from build123d import *

# Parameters (mm, degrees)
F0_R      = 9.1
F1_DEPTH  = 20
F2_W      = 10
F2_H      = 17
F3_DEPTH  = 30
F4_W      = 10
F4_H      = 28
F5_DEPTH  = 25.4
F6_R      = 3
F7_R      = 1.99999
F8_R      = 2.5527
F9_DEPTH  = 7.001
F10_R     = 1.35255
F11_DEPTH = 3.6831519111


# Not quite as in the source:
# - a fillet or chamfer is up to 0.001 mm smaller than in the source, because OpenCascade refuses the exact size


with BuildPart() as f1:
    # F0 (on Top) → F1 (new body)
    with BuildSketch(Plane.XY):
        with BuildLine():
            ThreePointArc((2.8507034294, -10.1056167529), (8.3720483159, -6.3370976792), (10.5, 0))
            ThreePointArc((10.5, 0), (9.0208092763, 5.3735463151), (5, 9.2330926563))
            Line((5, 9.2330926563), (-5, 9.2330926563))
            ThreePointArc((-5, 9.2330926563), (-10.4357465707, -1.1598247764), (-2.8507034294, -10.1056167529))
            Line((-2.8507034294, -10.1056167529), (2.8507034294, -10.1056167529))
        make_face()
        Circle(F0_R, mode=Mode.SUBTRACT)
        with BuildLine():
            Line((-5, 9.2330926563), (5, 9.2330926563))
            ThreePointArc((5, 9.2330926563), (0, 10.5), (-5, 9.2330926563))
        make_face()
        with BuildLine():
            ThreePointArc((-5, 9.2330926563), (0, 10.5), (5, 9.2330926563))
            Line((5, 9.2330926563), (5, 26.2330926563))
            Line((5, 26.2330926563), (-5, 26.2330926563))
            Line((-5, 26.2330926563), (-5, 9.2330926563))
        make_face()
        with BuildLine():
            Line((2.8507034294, -12.6810744405), (2.8507034294, -10.1056167529))
            ThreePointArc((2.8507034294, -10.1056167529), (0, -10.5), (-2.8507034294, -10.1056167529))
            Line((-2.8507034294, -10.1056167529), (-2.8507034294, -12.6810744405))
            Line((-2.8507034294, -12.6810744405), (2.8507034294, -12.6810744405))
        make_face()
        with BuildLine():
            ThreePointArc((-2.8507034294, -10.1056167529), (0, -10.5), (2.8507034294, -10.1056167529))
            Line((2.8507034294, -10.1056167529), (-2.8507034294, -10.1056167529))
        make_face()
    extrude(amount=F1_DEPTH)

    # F2 (on face) → F3 (join)
    with BuildSketch(Plane.XY.offset(20)):
        with Locations((0, 17.7330926563)):
            Rectangle(F2_W, F2_H)
    extrude(amount=F3_DEPTH)

    # F4 (on face) → F5 (cut)
    with BuildSketch(Plane.YZ.offset(5)):
        with Locations((14.2330926563, 36)):
            Rectangle(F4_W, F4_H)
    extrude(amount=-F5_DEPTH, mode=Mode.SUBTRACT)

    # F6
    f6_edges = [f1.edges().sort_by_distance(p)[0] for p in [
        (5, 9.233093, 10),
        (-5, 9.233093, 10),
        (-5, 22.733093, 50),
        (5, 22.733093, 50),
        (2.850703, -10.105617, 10),
        (-2.850703, -10.105617, 10),
    ]]
    fillet(f6_edges, radius=F6_R)

    # F7 (radius 2 in the source; OpenCascade refuses exactly that, so slightly less here)
    f7_edges = [f1.edges().sort_by_distance(p)[0] for p in [
        (0, 9.233093, 22),
        (0, 19.233093, 22),
    ]]
    fillet(f7_edges, radius=F7_R)

    # F8 (on face) → F9 (cut, through all)
    with BuildSketch(Plane.XZ.offset(-19.2330926563)):
        with Locations((0, 44)):
            Circle(F8_R)
        with Locations((0, 30)):
            Circle(F8_R)
    extrude(amount=-F9_DEPTH, mode=Mode.SUBTRACT)

    # F10 (on face) → F11 (cut, through all)
    with BuildSketch(Plane.XZ.offset(12.6810744405)):
        with Locations((0, 16)):
            Circle(F10_R)
        with Locations((0, 4)):
            Circle(F10_R)
    extrude(amount=-F11_DEPTH, mode=Mode.SUBTRACT)


solid = f1.part
Part model, mm, in its own coordinate system. A direction names the side the tool comes from. Give positions to 0.01 mm unless a question says otherwise; leave off trailing zeros. Order: outer loops, then holes, each group sorted by start corner. A loop starts at its lowest first (then second) coordinate and runs counter-clockwise, first axis right, second up. Notation, with made-up numbers: (-25, 54.25) -> (17, 54.25) arc R7 ccw to (17, 65.25) -> close; hole circle Ø11 at (89.5, -40). An arc over 180 degrees is marked (long way). Use one line per item in the form item = value.
(1) Flat gauge pins, fed straight in: P1, Ø4, axis at y = 5.5, z = 7, coming from the +X side; P2, Ø6, axis at x = 0, z = 44, coming from the -Y side; P3, Ø10, axis at x = -8, y = 4, coming from the +Z side. Where does each tip first touch, or does it go through?
Solution:
P1 = 9.9
P2 = 19.23
P3 = 20
(2) Pull direction X, two halves, no side cores. Call faces 4 (the face through (0, 14, 22)), 5 (the face through (-1.973, -8.884, 9.86)), 6 (the face through (-10.468, -0.824, 9.86)): +X half, -X half, draft (parallel to the pull), parting line (faces both ways), or undercut.
Solution:
face_4 = draft
face_5 = undercut
face_6 = -X half
(3) Saw through at B-B (x = 0). Count the separate pieces of the cut face and the enclosed holes in it, then the cut area to 3 significant figures.
Solution:
separate_pieces = 6
enclosed_holes = 0
area = 553 mm²
(4) Saw through at C-C (y = -3). Write the cut outline in (x, z).
Solution:
outline = (-10.06, 0) -> (-8.59, 0) -> (-8.59, 20) -> (-10.06, 20) -> close; (8.59, 0) -> (10.06, 0) -> (10.06, 20) -> (8.59, 20) -> close
(5) Saw through at A-A (z = 30). Write the cut outline in (x, y), then the cut area to 3 significant figures.
Solution:
outline = (-5, 19.23) -> (-2.55, 19.23) -> (-2.55, 26.23) -> (-5, 26.23) -> close; (2.55, 19.23) -> (5, 19.23) -> (5, 26.23) -> (2.55, 26.23) -> close
area = 34.3 mm²
(6) Drill centre lines: line 1 (Z direction, x = 0, y = 23.75); line 2 (Z direction, x = 0, y = -10.2); line 3 (Y direction, x = 4.25, z = 28.5). Where is each one in solid material? Low to high. Write a range as from..to.
Solution:
line_1 = 0..27.45, 32.55..41.45, 46.55..50
line_2 = 0..2.65, 5.35..14.65, 17.35..20
line_3 = 19.23..26.23
(7) Saw through at D-D (y = 23). Write the cut outline in (x, z), then the cut area to 3 significant figures.
Solution:
outline = (-5, 0) -> (5, 0) -> (5, 47) arc R3 ccw to (2, 50) -> (-2, 50) arc R3 ccw to (-5, 47) -> close; hole circle Ø5.11 at (0, 30); hole circle Ø5.11 at (0, 44)
area = 455 mm²
(8) Tool access for faces 1 (the face through (-0.29, -10.86, 2.68)), 2 (the face through (0, 19.233, 37)), 3 (the face through (-0.553, 22.684, 27.508)): list every direction of +Z, -Z, +X, -X, +Y, -Y with a clear straight run to the whole face (end or side of a thin tool).
Solution:
face_1 = -Y
face_2 = +Z, +X, -X, -Y
face_3 = +Y, -Y
